For this review, take the finished solid that the model builds, in its own axes (mm). A direction names the side the tool comes from. Give positions to 0.01 mm unless a question says otherwise; leave off trailing zeros. Write each loop counter-clockwise with the first axis right and the second up, starting at its lowest first coordinate (ties: lowest second). Pieces come first, ordered by that corner, then holes. Notation, with made-up numbers: (-23.5, 71.25) -> (29.5, 71.25) arc R17 ccw to (29.5, 100.25) -> close; hole circle Ø2 at (-38, -18.75). An arc over 180 degrees is marked (long way). Write item = value, one per line.
```python
from build123d import *

# Parameters (mm, degrees)
PAD_DEPTH         = 10
POCKET_DEPTH      = 20.903093
POCKET_DEPTH_BACK = -1.903093
SKETCH002_R       = 2.75
HOLE_DEPTH        = 25
FILLET_R          = 1


with BuildPart() as part:
    # Sketch → Pad (new body)
    with BuildSketch(Plane.XY):
        Polygon((0, 0), (19, 0), (20.902093, 10.787306), (20.114247, 10.926225), (18.32872, 0.8), (0.67128, 0.8), (-1.114247, 10.926225), (-1.902093, 10.787306), align=None)
    extrude(amount=PAD_DEPTH)

    # Sketch001 (on DatumPlane) → Pocket (cut, two sides)
    with BuildSketch(Plane(origin=(0, 0.8, 0), x_dir=(0, -1, 0), z_dir=(-1, 0, 0))) as pocket_sk:
        Polygon((-2.732161, 10.911916), (-2.732161, 7.99998), (-9.228047, 7.99998), (-9.832161, 7.576975), (-9.832161, 2.015372), (-9.381735, 1.69998), (-2.985139, 1.69998), (-2.985139, -3.596473), (-13.732095, -3.596473), (-13.732095, 10.911916), align=None)
    extrude(amount=-POCKET_DEPTH, mode=Mode.SUBTRACT)
    extrude(pocket_sk.sketch, amount=-POCKET_DEPTH_BACK, mode=Mode.SUBTRACT)

    # Sketch002 (on Face21 of Pocket) → Hole (cut)
    with BuildSketch(Plane(origin=(0, 0.8, 0), x_dir=(-1, 0, 0), z_dir=(0, 1, 0))):
        with Locations((-10.071387, 5.216614)):
            Circle(SKETCH002_R)
    extrude(amount=-HOLE_DEPTH, mode=Mode.SUBTRACT)

    # Fillet
    fillet_edges = [part.edges().sort_by_distance(p)[0] for p in [
        (19, 0, 5),
        (0, 0, 5),
        (0.67128, 0.8, 5),
        (18.32872, 0.8, 5),
    ]]
    fillet(fillet_edges, radius=FILLET_R)


solid = part.part
```
(1) For pin 1 (0.6 mm diameter, centred on x = 19.5, y = 8.5, fed in from -Z); pin 2 (3 mm diameter, centred on y = 8.5, z = 5, fed in from +X); pin 3 (2 mm diameter, centred on x = 18, y = 8.5, fed in from -Z); pin 4 (1 mm diameter, centred on x = 19.5, y = 7, fed in from +Z), all flat-tipped, find the tip position at first contact; note any pin that passes through.
Answers below:
pin_1 = 1.7
pin_2 = 20.76
pin_3 = through
pin_4 = 8
(2) To check wall thickness, follow probe 1 along X at (y, z) = (3.75, 3.5); probe 2 along Y at (x, z) = (14, 3); probe 3 along X at (y, z) = (5, 2.25). State the ranges of each line that lie inside material, in increasing order.
Answers below:
probe_1 = -0.66 to 0.15, 18.85 to 19.66
probe_2 = 0 to 0.8
probe_3 = -0.88 to -0.07, 19.07 to 19.88
(3) Tool access review of faces 1 (the face through (20, 7, 1.7)), 2 (the face through (0.875, 1.028, 5.07)), 3 (the face through (0, 3.532, 9)): name each direction out of +Z, -Z, +X, -X, +Y, -Y from which nothing blocks a thin tool from reaching the whole face with its end or side.
Answers below:
face_1 = -Z, +X, -X, +Y
face_2 = +Z, -Z, +Y
face_3 = +Z, +X, -X, +Y
(4) Take a section at D-D (z = 7.25). Write out the cut boundary in (x, y).
Answers below:
outline = (-1.87, 10.63) -> (-0.15, 0.83) arc R1 ccw to (0.84, 0) -> (8.22, 0) -> (8.22, 0.8) -> (1.51, 0.8) arc R1 cw to (0.53, 1.63) -> (-1.06, 10.63) -> close; (11.92, 0) -> (18.16, 0) arc R1 ccw to (19.15, 0.83) -> (20.87, 10.63) -> (20.06, 10.63) -> (18.47, 1.63) arc R1 cw to (17.49, 0.8) -> (11.92, 0.8) -> close
(5) Take a section at B-B (x = 12.5). Write out the cut boundary in (y, z), plus the area to 3 significant figures.
Answers below:
outline = (0, 0) -> (0.8, 0) -> (0.8, 3.93) -> (0, 3.93) -> close; (0, 6.51) -> (0.8, 6.51) -> (0.8, 10) -> (0, 10) -> close
area = 5.94 mm^2
(6) Take a section at C-C (y = 9). Write out the cut boundary in (x, z).
Answers below:
outline = (-1.59, 1.7) -> (-0.77, 1.7) -> (-0.77, 8) -> (-1.59, 8) -> close; (19.77, 1.7) -> (20.59, 1.7) -> (20.59, 8) -> (19.77, 8) -> close
(7) Take a section at A-A (z = 8.5). Write out the cut boundary in (x, y).
Answers below:
outline = (-0.62, 3.53) -> (-0.15, 0.83) arc R1 ccw to (0.84, 0) -> (18.16, 0) arc R1 ccw to (19.15, 0.83) -> (19.62, 3.53) -> (18.81, 3.53) -> (18.47, 1.63) arc R1 cw to (17.49, 0.8) -> (1.51, 0.8) arc R1 cw to (0.53, 1.63) -> (0.19, 3.53) -> close
